Part print with two shaded views. Sizes in mm from the minimum x, y, z corner. A direction names the side the tool comes from. Round coordinates to 2 decimals unless told otherwise and drop trailing zeros. Order: outer loops, then holes, each group sorted by start corner. A loop starts at its lowest first (then second) coordinate and runs counter-clockwise, first axis right, second up. Notation, with made-up numbers: (19.5, 42) -> (72.5, 42) arc R20 ccw to (72.5, 47) -> close; hole circle Ø2 at (1.5, -16.75). An arc over 180 degrees is marked (long way). Put each result on its own line as item: value. Start each with the question number.
Q1. Cut at B-B, the plane z = 6. List the corners of the cut face in (x, y).
Q2. Cut at A-A, the plane z = 12.7. List the corners of the cut face in (x, y) (1 decimal), and give its area (3 significant figures).
Q3. Pull direction X, two halves, no side cores. Call the marked faces 1, 2 and 3: released by +X, released by -X, zero draft, split by the parting line, or undercut.
Q4. Flat gauge pins, fed straight in: P1, Ø6.5, axis at x = 11, z = 11, coming from the +Y side; P2, Ø1, axis at y = 4, z = 21.5, coming from the -X side. Where does each tip first touch, or does it go through?
Q5. Cut at D-D, the plane x = 22.75. List the corners of the cut face in (y, z).
Q6. 3-axis set-ups, long thin cutter, end or side, ignore diameter. For the marked faces 4, 5 and 6: which of +Z, -Z, +X, -X, +Y, -Y reach the whole face in a straight line?
Q7. Probe L1, parallel to Y at x = 24.6, z = 12.7 (1 decimal); L2, parallel to X at y = 19, z = 6.75; L3, parallel to Z at x = 12.25, y = 10. List the from-to ranges inside material, lowest first.
Q8. Cut at C-C, the plane y = 21. List the corners of the cut face in (x, z), and give its area (3 significant figures).
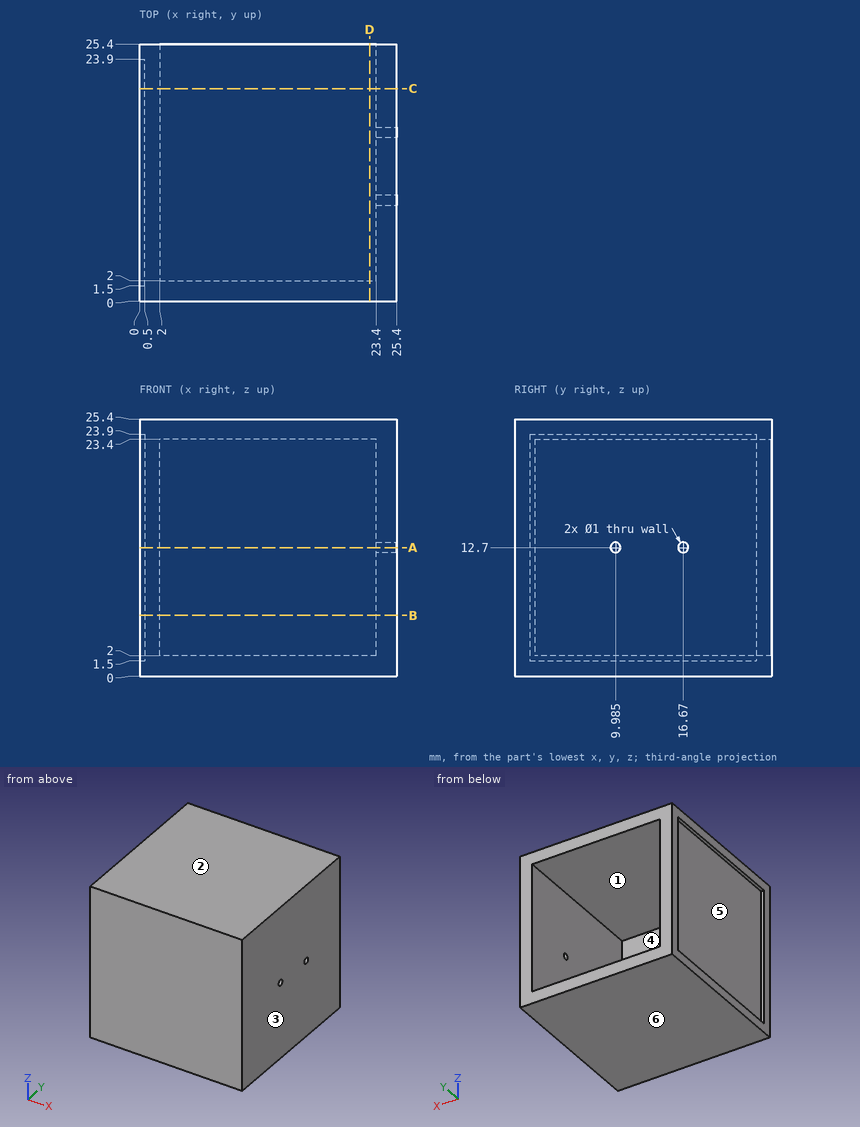
Ans:
1. outline: (0, 0) -> (25.4, 0) -> (25.4, 25.4) -> (23.4, 25.4) -> (23.4, 2) -> (2, 2) -> (2, 25.4) -> (0, 25.4) -> (0, 23.9) -> (0.5, 23.9) -> (0.5, 1.5) -> (0, 1.5) -> close
2. outline: (0, 0) -> (25.4, 0) -> (25.4, 9.5) -> (23.4, 9.5) -> (23.4, 2) -> (2, 2) -> (2, 25.4) -> (0, 25.4) -> (0, 23.9) -> (0.5, 23.9) -> (0.5, 1.5) -> (0, 1.5) -> close; (23.4, 10.5) -> (25.4, 10.5) -> (25.4, 16.2) -> (23.4, 16.2) -> close; (23.4, 17.2) -> (25.4, 17.2) -> (25.4, 25.4) -> (23.4, 25.4) -> close
2. area: 129 mm^2
3. face 1: undercut
3. face 2: zero draft
3. face 3: released by +X
4. P1: stops at y = 2
4. P2: stops at x = 0.5
5. outline: (0, 0) -> (25.4, 0) -> (25.4, 2) -> (2, 2) -> (2, 23.4) -> (25.4, 23.4) -> (25.4, 25.4) -> (0, 25.4) -> close
6. face 4: +Y
6. face 5: -X
6. face 6: -Z, +X, -X, +Y, -Y
7. L1: y = 0 to 9.5, 10.5 to 16.2, 17.2 to 25.4
7. L2: x = 0.5 to 2, 23.4 to 25.4
7. L3: z = 0 to 2, 23.4 to 25.4
8. outline: (0, 0) -> (25.4, 0) -> (25.4, 25.4) -> (0, 25.4) -> (0, 23.9) -> (0.5, 23.9) -> (0.5, 1.5) -> (0, 1.5) -> close; hole (2, 2) -> (23.4, 2) -> (23.4, 23.4) -> (2, 23.4) -> close
8. area: 176 mm^2
